The drawing under review shows one solid part. Ordinate dimensions are in mm from its lowest x, y, z. Coordinates: 2 decimals unless noted, no trailing zeros. Order: outer loops, then holes, each group sorted by start corner. A loop starts at its lowest first (then second) coordinate and runs counter-clockwise, first axis right, second up. Notation, with made-up numbers: (47.25, -37) -> (79.25, -37) arc R35 ccw to (79.25, -2) -> close; hole circle Ø6 at (-40, -35.75). An arc over 180 degrees is marked (long way). Put each result on its own line as item: value.
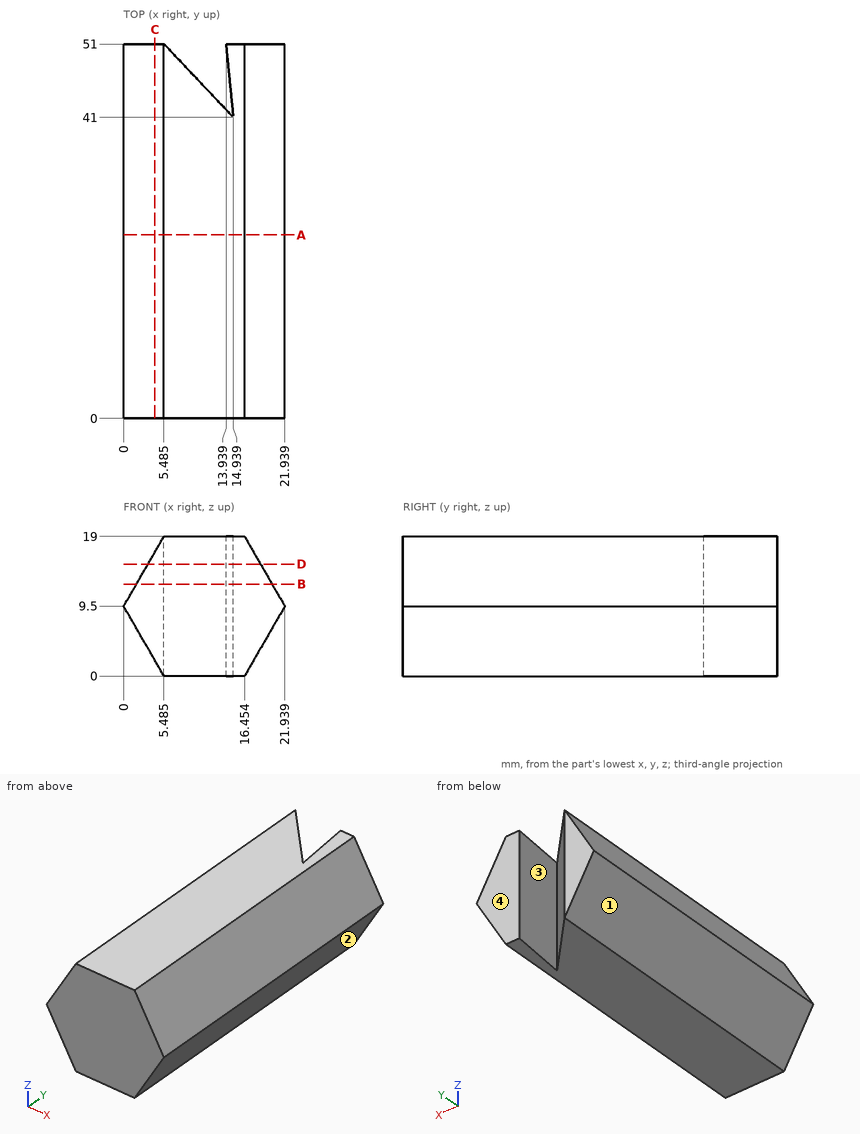
Item 1: Consider section D-D on z = 15.25. Write out the cut boundary in (x, y) (1 decimal), and give its area (3 significant figures).
Answers below:
outline: (3.3, 0) -> (18.6, 0) -> (18.6, 51) -> (13.9, 51) -> (14.9, 41) -> (5.5, 51) -> (3.3, 51) -> close
area: 738 mm^2
Item 2: Consider section C-C on x = 4.25. Write out the cut boundary in (y, z).
Answers below:
outline: (0, 2.14) -> (51, 2.14) -> (51, 16.86) -> (0, 16.86) -> close
Item 3: Mouldability with a two-part tool opening along X and no side actions: class the marked faces 1, 2, 3 and 4 as +X half, -X half, draft (parallel to the pull), parting line (faces both ways), or undercut.
Answers below:
face 1: -X half
face 2: +X half
face 3: undercut
face 4: draft
Item 4: Consider section B-B on z = 12.5. Write out the cut boundary in (x, y) (1 decimal), and give its area (3 significant figures).
Answers below:
outline: (1.7, 0) -> (20.2, 0) -> (20.2, 51) -> (13.9, 51) -> (14.9, 41) -> (5.5, 51) -> (1.7, 51) -> close
area: 900 mm^2
Item 5: For pin 1 Ø1.5 at (x, y) = (3.5, 24.5) entering from +Z; pin 2 Ø8 at (y, z) = (5.5, 14) entering from -X, all flat-tipped, find the tip position at first contact; note any pin that passes through.
Answers below:
pin 1: z = 16.86
pin 2: x = 0.29
Item 6: For line 1 (X direction, y = 45, z = 12.5) (1 decimal); line 2 (X direction, y = 31, z = 1.5); line 3 (Y direction, x = 10.25, z = 7), list the stretches that pass through material, from the lowest coordinate up. Write a range as from..to.
Answers below:
line 1: 1.7..11.2, 14.5..20.2
line 2: 4.62..17.32
line 3: 0..45.96
Item 7: Consider section A-A on y = 25. Write out the cut boundary in (x, z) (1 decimal), and give its area (3 significant figures).
Answers below:
outline: (0, 9.5) -> (5.5, 0) -> (16.5, 0) -> (21.9, 9.5) -> (16.5, 19) -> (5.5, 19) -> close
area: 313 mm^2
